Input: part model. Units: mm. Frame: model coordinates. Face numbers are marked on the shaded views. A direction names the side the tool comes from. Give positions to 0.01 mm unless a question says otherwise; leave off trailing zeros. One line per question, with ' | ' between items.
from build123d import *

# Parameters (mm, degrees)
F1_DEPTH = 30
F2_DEPTH = 2
F3_SIZE  = 1.99999
F5_DEPTH = 25
F6_SIZE  = 0.99999


# Not quite as in the source:
# - a fillet or chamfer is up to 0.001 mm smaller than in the source, because OpenCascade refuses the exact size


with BuildPart() as f1:
    # F0 (on Top) → F1 (new body)
    with BuildSketch(Plane.XY):
        Polygon((17.5, 20), (-17.5, 20), (-32.5, 0), (-17.5, -20), (17.5, -20), (32.5, 0), align=None)
        Polygon((16.5, -18), (-16.5, -18), (-30, 0), (-16.5, 18), (16.5, 18), (30, 0), align=None, mode=Mode.SUBTRACT)
    extrude(amount=F1_DEPTH)

    # F0 (on Top) → F2 (join)
    with BuildSketch(Plane.XY):
        Polygon((-45, 0), (-22.5, -30), (22.5, -30), (45, 0), (22.5, 30), (-22.5, 30), align=None)
        Polygon((-32.5, 0), (-17.5, 20), (17.5, 20), (32.5, 0), (17.5, -20), (-17.5, -20), align=None, mode=Mode.SUBTRACT)
    extrude(amount=F2_DEPTH)

    # F3 (size 2 in the source; OpenCascade refuses exactly that, so slightly less here)
    f3_edges = [f1.edges().sort_by_distance(p)[0] for p in [
        (-25, 10, 30),
        (0, 20, 30),
        (25, 10, 30),
        (25, -10, 30),
        (0, -20, 30),
        (-25, -10, 30),
        (0, -30, 2),
        (33.75, -15, 2),
        (33.75, 15, 2),
        (-33.75, -15, 2),
        (-33.75, 15, 2),
        (0, 30, 2),
    ]]
    chamfer(f3_edges, length=F3_SIZE)

    # F4 (on Top) → F5 (join)
    with BuildSketch(Plane.XY):
        Polygon((-17.1708203932, -17.105572809), (-16.5, -18), (-15.3819660113, -18), (-10.8819660113, -9), (10.8819660113, -9), (15.3819660113, -18), (16.5, -18), (17.1708203932, -17.105572809), (12.6708203932, -8.105572809), (18, -1), (29.25, -1), (30, 0), (29.25, 1), (18, 1), (12.6708203932, 8.105572809), (17.1708203932, 17.105572809), (16.5, 18), (15.3819660113, 18), (10.8819660113, 9), (-10.8819660113, 9), (-15.3819660113, 18), (-16.5, 18), (-17.1708203932, 17.105572809), (-12.6708203932, 8.105572809), (-18, 1), (-29.25, 1), (-30, 0), (-29.25, -1), (-18, -1), (-12.6708203932, -8.105572809), align=None)
        Polygon((-11, -7), (-16.25, 0), (-11, 7), (11, 7), (16.25, 0), (11, -7), align=None, mode=Mode.SUBTRACT)
    extrude(amount=F5_DEPTH)

    # F6 (size 1 in the source; OpenCascade refuses exactly that, so slightly less here)
    f6_edges = [f1.edges().sort_by_distance(p)[0] for p in [
        (-23.625, -1, 25),
        (-23.625, 1, 25),
        (-15.33541, -4.552786, 25),
        (-13.625, -3.5, 25),
        (-13.625, 3.5, 25),
        (-15.33541, 4.552786, 25),
        (-14.92082, 12.605573, 25),
        (-13.131966, 13.5, 25),
        (0, 7, 25),
        (0, 9, 25),
        (0, -9, 25),
        (0, -7, 25),
        (-13.131966, -13.5, 25),
        (-14.92082, -12.605573, 25),
        (14.92082, -12.605573, 25),
        (13.131966, -13.5, 25),
        (15.33541, -4.552786, 25),
        (13.625, -3.5, 25),
        (23.625, -1, 25),
        (23.625, 1, 25),
        (15.33541, 4.552786, 25),
        (13.625, 3.5, 25),
        (14.92082, 12.605573, 25),
        (13.131966, 13.5, 25),
    ]]
    chamfer(f6_edges, length=F6_SIZE)


solid = f1.part
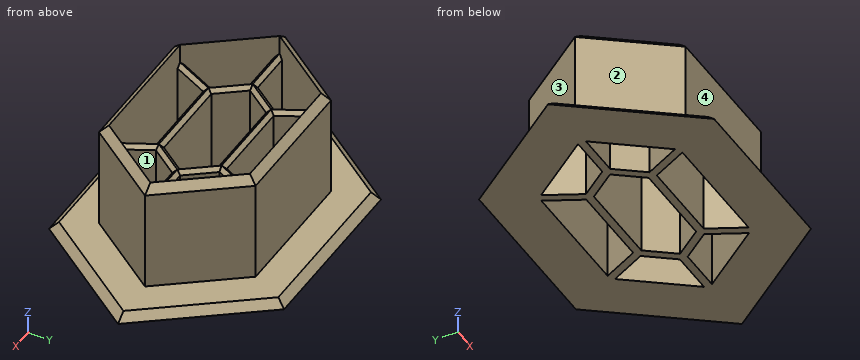
1. Ray query, line 1 along Y through (x, z) = (10, 2.5); line 2 along X through (y, z) = (-13.5, 12.25) (3 decimals); line 3 along X through (y, z) = (2, 13.5). Return the intervals inside material, ascending. Write a range as from..to.
Determined:
line 1: y = -20..-18, -9..-7, 7..9, 18..20 | line 2: x = -22.375..-19.875, -15.368..-13.132, 13.132..15.368, 19.875..22.375 | line 3: x = -31..-28.5, -17.25..-14.75, 14.75..17.25, 28.5..31
2. Section query A-A (y = -13). Count the separate pieces of the cut face and the enclosed holes in it, then the cut area to 3 significant figures.
Determined:
separate pieces: 4 | enclosed holes: 0 | area: 300 mm2
3. Pin query (flat end, axial travel): P1, Ø5.5, axis at x = 22, z = 18, coming from the -Y side; P2, Ø6, axis at x = 15.5, y = 20, coming from the +Z side; P3, Ø15, axis at x = -1.5, z = 12, coming from the -Y side; P4, Ø9, axis at x = -23.5, z = 13.5, coming from the -Y side. Return the tip coordinate at first contact, or that it passes through.
Determined:
P1: stops at y = -17.67 | P2: stops at z = 30 | P3: stops at y = -20 | P4: stops at y = -18
4. Reachability of the marked faces 1, 2, 3 and 4 from +Z, -Z, +X, -X, +Y, -Y: full face, straight path, thin tool, end or side. Return the list, or none.
Determined:
face 1: +Z, -Z | face 2: +Z, -X, -Y | face 3: +Z, -X, +Y | face 4: +Z, +X, -X, -Y
